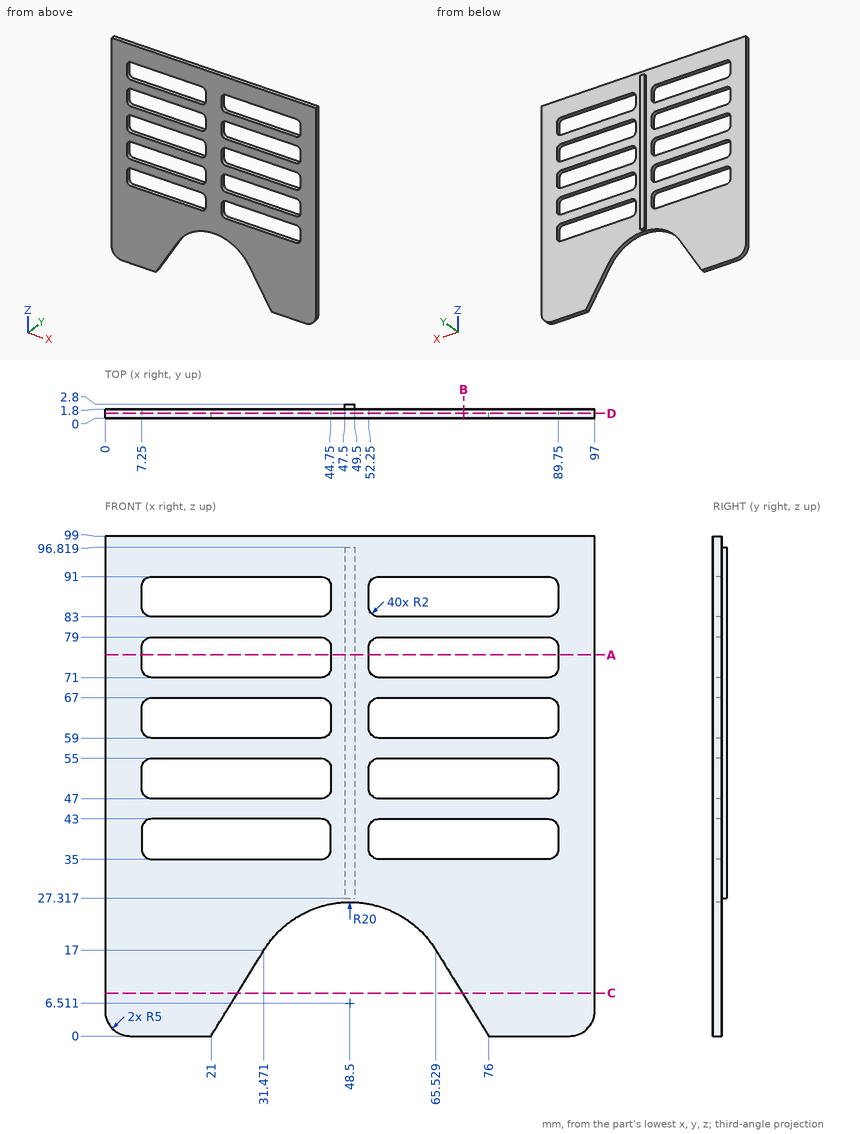
Can you work these out from the drawing? Everything is in mm from the part's minimum corner. Round coordinates to 2 decimals unless told otherwise and drop trailing zeros. Loops run counter-clockwise (first coordinate to the right, second up) from the corner with the lowest first, then second, coordinate; pieces in that order, holes last. Notation, with made-up numbers: (79.25, 25) - (126.25, 25) arc R10 ccw to (126.25, 40) - close; hole circle Ø4 at (21.5, 69). An arc over 180 degrees is marked (long way). Answer in a Markdown table with one row per item. Add a question column.
Q1. For pin 1 Ø6 at (x, z) = (53, 59.5) entering from +Y, with a flat end and sliding along its axis, tell me the tip position at first contact or that it passes through.
Q2. I want a section at D-D on y = 0.95. Count the separate pieces of the cut face and the enclosed holes in it, and give its area (3 significant figures).
Q3. I want a section at A-A on z = 75.5. List the corners of the cut face in (x, y) for me.
Q4. I want a section at B-B on x = 71. List the corners of the cut face in (y, z) for me.
Q5. I need wall thicknesses on L1, parallel to X at y = 0.7, z = 49; L2, parallel to Z at x = 82.5, y = 0.35; L3, parallel to Z at x = 64, y = 0.8. Which ranges of each line are inside material? Lowest first, please.
Q6. I want a section at C-C on z = 8.5. List the corners of the cut face in (x, y) for me (1 decimal).
A:
| question | item | result |
|---|---|---|
| 1 | pin 1 | y = 1.8 |
| 2 | separate pieces | 1 |
| 2 | enclosed holes | 10 |
| 2 | area | 5,640 mm^2 |
| 3 | outline | (0, 0) - (7.25, 0) - (7.25, 1.8) - (0, 1.8) - close; (44.75, 0) - (52.25, 0) - (52.25, 1.8) - (49.5, 1.8) - (49.5, 2.8) - (47.5, 2.8) - (47.5, 1.8) - (44.75, 1.8) - close; (89.75, 0) - (97, 0) - (97, 1.8) - (89.75, 1.8) - close |
| 4 | outline | (0, 8.12) - (1.8, 8.12) - (1.8, 35) - (0, 35) - close; (0, 43) - (1.8, 43) - (1.8, 47) - (0, 47) - close; (0, 55) - (1.8, 55) - (1.8, 59) - (0, 59) - close; (0, 67) - (1.8, 67) - (1.8, 71) - (0, 71) - close; (0, 79) - (1.8, 79) - (1.8, 83) - (0, 83) - close; (0, 91) - (1.8, 91) - (1.8, 99) - (0, 99) - close |
| 5 | L1 | 0 to 7.25, 44.75 to 52.25, 89.75 to 97 |
| 5 | L2 | 0 to 35, 43 to 47, 55 to 59, 67 to 71, 79 to 83, 91 to 99 |
| 5 | L3 | 19.15 to 35, 43 to 47, 55 to 59, 67 to 71, 79 to 83, 91 to 99 |
| 6 | outline | (0, 0) - (26.2, 0) - (26.2, 1.8) - (0, 1.8) - close; (70.8, 0) - (97, 0) - (97, 1.8) - (70.8, 1.8) - close |
